```python
from build123d import *

# Parameters (mm, degrees)
CROQUIS1_W              = 2.1
CROQUIS1_H              = 21.5
SALIENTE_EXTRUIR1_DEPTH = 1.5
REDONDEO1_R             = 10
CROQUIS2_W              = 3
CROQUIS2_H              = 17
SALIENTE_EXTRUIR2_DEPTH = 3
CROQUIS3_W              = 3
CROQUIS3_H              = 17
SALIENTE_EXTRUIR3_DEPTH = 3
REDONDEO2_R             = 10
REDONDEO3_R             = 10
CROQUIS5_W              = 21.447905668
CROQUIS5_H              = 38.241159468
CORTAR_EXTRUIR2_DEPTH   = 10
REDONDEO4_R             = 10
CORTAR_EXTRUIR3_DEPTH   = 10


with BuildPart() as part:
    # Croquis1 → Saliente-Extruir1 (new, symmetric)
    with BuildSketch(Plane(origin=(0, 0, 0), x_dir=(0, 0, -1), z_dir=(1, 0, 0))):
        Polygon((14, -12.5), (17, -12.5), (17, -4.5), (14, -4.5), (14, 4.5), (17, 4.5), (17, 12.5), (-10, 12.5), (-10, -12.5), align=None)
        Rectangle(CROQUIS1_W, CROQUIS1_H, mode=Mode.SUBTRACT)
    extrude(amount=SALIENTE_EXTRUIR1_DEPTH, both=True)

    # Redondeo1
    redondeo1_edges = [part.edges().sort_by_distance(p)[0] for p in [
        (0, -12.5, 10),
        (0, 12.5, 10),
    ]]
    fillet(redondeo1_edges, radius=REDONDEO1_R)

    # Croquis2 → Saliente-Extruir2 (add)
    with BuildSketch(Plane(origin=(0, 12.5, 0), x_dir=(1, 0, 0), z_dir=(0, 1, 0))):
        with Locations((0, 8.5)):
            Rectangle(CROQUIS2_W, CROQUIS2_H)
    extrude(amount=SALIENTE_EXTRUIR2_DEPTH)

    # Croquis3 → Saliente-Extruir3 (add)
    with BuildSketch(Plane.XZ.offset(12.5)):
        with Locations((0, -8.5)):
            Rectangle(CROQUIS3_W, CROQUIS3_H)
    extrude(amount=SALIENTE_EXTRUIR3_DEPTH)

    # Redondeo2
    # the kernel refuses this fillet: 10 mm, written as the material it adds along each edge
    with BuildSketch(Plane(origin=(1.5, -12.5, 0), x_dir=(0, -1, 0), z_dir=(-1, 0, 0))) as redondeo2_piece_1:
        with BuildLine():
            CenterArc((8.038461538, 8.637934089), REDONDEO2_R, 205.587990121, 34.157222478)
            Line((-0.980769231, 4.318967044), (-1.161153846, 4.232587704))
            ThreePointArc((-1.161153846, 4.232587704), (-0.443308828, 2.17017369), (-0.2, 0))
            Line((-0.2, 0), (0, -0.2))
            ThreePointArc((0, -0.2), (1.5, -0.2), (2.899230769, -0.172758682))
            Line((2.899230769, -0.172758682), (3, 0))
        make_face()
    extrude(amount=3)
    with BuildSketch(Plane(origin=(1.5, 12.5, 0), x_dir=(0, 1, 0), z_dir=(-1, 0, 0))) as redondeo2_piece_2:
        with BuildLine():
            CenterArc((8.038461538, -8.637934089), REDONDEO2_R, 120.254787401, 34.157222478)
            Line((-0.980769231, -4.318967044), (-1.161153846, -4.232587704))
            ThreePointArc((-1.161153846, -4.232587704), (-0.443308828, -2.17017369), (-0.2, 0))
            Line((-0.2, 0), (0, 0.2))
            ThreePointArc((0, 0.2), (1.5, 0.2), (2.899230769, 0.172758682))
            Line((2.899230769, 0.172758682), (3, 0))
        make_face()
    extrude(amount=3)

    # Redondeo3
    redondeo3_edges = [part.edges().sort_by_distance(p)[0] for p in [
        (0, 15.5, 0),
        (0, -15.5, 0),
    ]]
    fillet(redondeo3_edges, radius=REDONDEO3_R)

    # Croquis5 → Cortar-Extruir2 (cut)
    with BuildSketch(Plane(origin=(1.5, 0, 0), x_dir=(0, 0, -1), z_dir=(1, 0, 0))):
        with Locations((-14.773952834, -0.867042995)):
            Rectangle(CROQUIS5_W, CROQUIS5_H)
    extrude(amount=-CORTAR_EXTRUIR2_DEPTH, mode=Mode.SUBTRACT)

    # Redondeo4
    # the kernel refuses this fillet: 10 mm, written as the material it takes off along each edge
    with BuildSketch(Plane(origin=(-13.099738715, 11.653031847, 4.05), x_dir=(0, 0.5631802476031196, -0.8263340781485954), z_dir=(1, 0, 0))) as redondeo4_piece_1:
        with BuildLine():
            CenterArc((5.650243293, -9.465906235), REDONDEO4_R, 108.810422247, 36.913558107)
            Line((-2.613097489, -3.834103759), (-2.778364304, -3.72146771))
            Line((-2.778364304, -3.72146771), (-0.165266816, 0.11263605))
            Line((-0.165266816, 0.11263605), (0.024258644, 0.198523344))
            ThreePointArc((0.024258644, 0.198523344), (1.212932207, 0.126167209), (2.361376837, 0.189318125))
            Line((2.361376837, 0.189318125), (2.425864415, 0))
        make_face()
    extrude(amount=26.19947743, mode=Mode.SUBTRACT)
    with BuildSketch(Plane(origin=(-13.099738715, -11.653031847, 4.05), x_dir=(0, 1, 0), z_dir=(1, 0, 0))) as redondeo4_piece_2:
        with BuildLine():
            CenterArc((4.639895486, -10), REDONDEO4_R, 90, 36.913558107)
            Line((-1.366198922, -2.004574435), (-1.48632081, -1.844665924))
            ThreePointArc((-1.48632081, -1.844665924), (-0.787355725, -0.931232338), (-0.177708594, 0.091758682))
            Line((-0.177708594, 0.091758682), (0, 0.2))
            Line((0, 0.2), (4.639895486, 0.2))
            Line((4.639895486, 0.2), (4.639895486, 0))
        make_face()
    extrude(amount=26.19947743, mode=Mode.SUBTRACT)

    # Croquis6 → Cortar-Extruir3 (cut)
    with BuildSketch(Plane(origin=(1.5, 0, 0), x_dir=(0, 0, -1), z_dir=(1, 0, 0))):
        Polygon((14, 1.5), (11, 1.5), (11, 4), (8, 4), (8, 1.5), (6, 1.5), (6, -1.5), (8, -1.5), (8, -4), (11, -4), (11, -1.5), (14, -1.5), align=None)
    extrude(amount=-CORTAR_EXTRUIR3_DEPTH, mode=Mode.SUBTRACT)


solid = part.part
```
Geometry check sheet. Reference: the model listing, model coordinates, mm. A direction names the side the tool comes from. Round coordinates to 2 decimals unless told otherwise and drop trailing zeros. Loops run counter-clockwise (first coordinate to the right, second up) from the corner with the lowest first, then second, coordinate; pieces in that order, holes last. Notation, with made-up numbers: M 3,88.25 L 52,88.25 A8 cw 52,93.25 Z; hole C -39.75,-33.75 d5. An arc over 180 degrees is marked long. Return JSON: item names as keys, results as strings. Group by question number.
(1) Mould release check, pull along Z, two halves, no side actions. Record for faces 4 (the face through (0, -3, -8)), 5 (the face through (0, 10, -17)), 6 (the face through (0, -1.5, -12)): pulls with the +Z half, pulls with the -Z half, needs draft (parallel to the pull), parting line crosses it, or undercut.
(2) Set-up check for faces 1 (the face through (0, 1.5, -7)), 2 (the face through (0, -3, -11)), 3 (the face through (1.5, 0, -4)): record each of +Z, -Z, +X, -X, +Y, -Y from which the full face is reachable in a straight line by a thin tool's end or side.
(3) Section check B-B, the plane z = -9.5. Enter the section's corners in (x, y), and give its area (3 significant figures).
(4) Section check A-A, the plane y = 2. Enter the section's corners in (x, z), and give its area (4 significant figures).
(5) Section check C-C, the plane x = -0.45. Enter the section's corners in (y, z).
(6) Section check D-D, the plane y = 8.5. Enter the section's corners in (x, z), and give its area (3 significant figures).
(7) Go/stop test with flat-tipped pins: pin 1 (0.9 mm diameter, centred on x = 0, y = 2.5, fed in from -Z); pin 2 (0.6 mm diameter, centred on x = -0.5, z = -0.5, fed in from +Y); pin 3 (1.7 mm diameter, centred on x = 0.5, z = 0.5, fed in from -Y). Record where each tip stops, or that it passes through.
(8) Scan lines: line 1 along Z through (x, y) = (-0.35, -5.5); line 2 along Z through (x, y) = (0.6, 1); line 3 along Y through (x, z) = (-0.55, -13.75). Record each from-to range of solid material in increasing order. Write a range as [from, to].
Data:
{
 "1": {"face 4": "undercut", "face 5": "pulls with the -Z half", "face 6": "needs draft"},
 "2": {"face 1": "-Z, +X, -X", "face 2": "+X, -X", "face 3": "+Z, -Z, +X, +Y, -Y"},
 "3": {"outline": "M -1.5,-15.5 L 1.5,-15.5 L 1.5,-4 L -1.5,-4 Z; M -1.5,4 L 1.5,4 L 1.5,15.5 L -1.5,15.5 Z", "area": "69.0 mm²"},
 "4": {"outline": "M -1.5,-14 L 1.5,-14 L 1.5,-11 L -1.5,-11 Z; M -1.5,-8 L 1.5,-8 L 1.5,-1.05 L -1.5,-1.05 Z; M -1.5,1.05 L 1.5,1.05 L 1.5,4.05 L -1.5,4.05 Z", "area": "38.85 mm²"},
 "5": {"outline": "M -15.5,-17 L -4.5,-17 L -4.5,-14 L -1.5,-14 L -1.5,-11 L -4,-11 L -4,-8 L -1.5,-8 L -1.5,-6 L 1.5,-6 L 1.5,-8 L 4,-8 L 4,-11 L 1.5,-11 L 1.5,-14 L 4.5,-14 L 4.5,-17 L 15.5,-17 L 15.5,-4.55 A10 ccw 13.02,2.05 A10 ccw 7.01,4.05 L -7.01,4.05 A10 ccw -13.02,2.05 A10 ccw -15.5,-4.55 Z; hole M -10.75,-1.05 L 10.75,-1.05 L 10.75,1.05 L -10.75,1.05 Z"},
 "6": {"outline": "M -1.5,-17 L 1.5,-17 L 1.5,-1.05 L -1.5,-1.05 Z; M -1.5,1.05 L 1.5,1.05 L 1.5,3.94 L -1.5,3.94 Z", "area": "56.5 mm²"},
 "7": {"pin 1": "z = -14", "pin 2": "y = 14.77", "pin 3": "y = -14.58"},
 "8": {"line 1": "[-17, -1.05], [1.05, 4.05]", "line 2": "[-6, -1.05], [1.05, 4.05]", "line 3": "[-15.5, -1.5], [1.5, 15.5]"}
}
